```python
from build123d import *

# Parameters (mm, degrees)
ESQUISSE1_W              = 200
ESQUISSE1_H              = 200
BOSS_EXTRU_1_DEPTH       = 50
ESQUISSE2_W              = 190
ESQUISSE2_H              = 190
ENL_V_MAT_EXTRU_1_DEPTH  = 40
ESQUISSE3_W              = 70
ESQUISSE3_H              = 24
ENL_V_MAT_EXTRU_2_DEPTH  = 10
ESQUISSE5_W              = 5
ESQUISSE5_H              = 18
ESQUISSE5_W_2            = 30
ESQUISSE5_H_2            = 14
ENL_V_MAT_EXTRU_3_DEPTH  = 6
ESQUISSE7_W              = 5
ESQUISSE7_H              = 14
ENL_V_MAT_EXTRU_5_DEPTH  = 6
ESQUISSE8_W              = 80
ESQUISSE8_H              = 5
ENL_V_MAT_EXTRU_6_DEPTH  = 10
ESQUISSE9_W              = 190
ESQUISSE9_H              = 5
BOSS_EXTRU_2_DEPTH       = 75
ESQUISSE11_W             = 50
ESQUISSE11_H             = 40
ESQUISSE11_W_2           = 40
ESQUISSE11_H_2           = 30
ENL_V_MAT_EXTRU_9_DEPTH  = 6
ESQUISSE12_R             = 5.86708194
ENL_V_MAT_EXTRU_10_DEPTH = 2
ESQUISSE13_W             = 20
ESQUISSE13_H             = 10
ENL_V_MAT_EXTRU_11_DEPTH = 5


with BuildPart() as part:
    # Esquisse1 → Boss.-Extru.1 (new body)
    with BuildSketch(Plane(origin=(0, 0, 0), x_dir=(1, 0, 0), z_dir=(0, 1, 0))):
        Rectangle(ESQUISSE1_W, ESQUISSE1_H)
    extrude(amount=BOSS_EXTRU_1_DEPTH)

    # Esquisse2 → Enlèv. mat.-Extru.1 (cut)
    with BuildSketch(Plane.XZ):
        Rectangle(ESQUISSE2_W, ESQUISSE2_H)
    extrude(amount=-ENL_V_MAT_EXTRU_1_DEPTH, mode=Mode.SUBTRACT)

    # Esquisse3 → Enlèv. mat.-Extru.2 (cut)
    with BuildSketch(Plane(origin=(0, 50, 0), x_dir=(1, 0, 0), z_dir=(0, 1, 0))):
        with Locations((0, 72)):
            Rectangle(ESQUISSE3_W, ESQUISSE3_H)
    extrude(amount=-ENL_V_MAT_EXTRU_2_DEPTH, mode=Mode.SUBTRACT)

    # Esquisse5 → Enlèv. mat.-Extru.3 (cut)
    with BuildSketch(Plane.XZ.offset(-40)):
        with Locations((37.5, -72)):
            Rectangle(ESQUISSE5_W, ESQUISSE5_H)
        with Locations((-20, -53)):
            Rectangle(ESQUISSE5_W_2, ESQUISSE5_H_2)
    extrude(amount=-ENL_V_MAT_EXTRU_3_DEPTH, mode=Mode.SUBTRACT)

    # Esquisse7 → Enlèv. mat.-Extru.5 (cut)
    with BuildSketch(Plane.XZ.offset(-40)):
        with Locations((-37.5, -53)):
            Rectangle(ESQUISSE7_W, ESQUISSE7_H)
    extrude(amount=-ENL_V_MAT_EXTRU_5_DEPTH, mode=Mode.SUBTRACT)

    # Esquisse8 → Enlèv. mat.-Extru.6 (cut)
    with BuildSketch(Plane.XZ.offset(-40)):
        with Locations((0, -40)):
            Rectangle(ESQUISSE8_W, ESQUISSE8_H)
    extrude(amount=-ENL_V_MAT_EXTRU_6_DEPTH, mode=Mode.SUBTRACT)

    # Esquisse9 → Boss.-Extru.2 (add)
    with BuildSketch(Plane(origin=(0, 0, 95), x_dir=(-1, 0, 0), z_dir=(0, 0, -1))):
        with Locations((0, 2.5)):
            Rectangle(ESQUISSE9_W, ESQUISSE9_H)
    extrude(amount=BOSS_EXTRU_2_DEPTH)

    # Esquisse11 → Enlèv. mat.-Extru.9 (cut)
    with BuildSketch(Plane.XZ.offset(-40)):
        with Locations((0, 16)):
            Rectangle(ESQUISSE11_W, ESQUISSE11_H)
        with Locations((0, 16)):
            Rectangle(ESQUISSE11_W_2, ESQUISSE11_H_2, mode=Mode.SUBTRACT)
    extrude(amount=-ENL_V_MAT_EXTRU_9_DEPTH, mode=Mode.SUBTRACT)

    # Esquisse12 → Enlèv. mat.-Extru.10 (cut)
    with BuildSketch(Plane(origin=(0, 50, 0), x_dir=(1, 0, 0), z_dir=(0, 1, 0))):
        with Locations(Location((0, -14.714419725, 0), (0, 0, 270))):
            Circle(ESQUISSE12_R)
        with BuildLine():
            ThreePointArc((3.657276348, -2.723473664), (12.412554836, -14.744243454), (3.657276348, -26.765013245))
            ThreePointArc((3.657276348, -26.765013245), (3.359240733, -32.427689923), (9.021917411, -32.725725538))
            ThreePointArc((9.021917411, -32.725725538), (20.02990103, -14.744243454), (9.021917411, 3.237238629))
            ThreePointArc((9.021917411, 3.237238629), (3.359240733, 2.939203014), (3.657276348, -2.723473664))
        make_face()
        with BuildLine():
            ThreePointArc((-4.091649632, -2.723473664), (-12.057804345, -14.744243454), (-4.091649632, -26.765013245))
            ThreePointArc((-4.091649632, -26.765013245), (-4.087653986, -32.721729891), (-10.044370632, -32.725725538))
            ThreePointArc((-10.044370632, -32.725725538), (-20.198964068, -14.893261262), (-10.044370632, 2.939203014))
            ThreePointArc((-10.044370632, 2.939203014), (-4.236671793, 3.084225175), (-4.091649632, -2.723473664))
        make_face()
        with BuildLine():
            ThreePointArc((13.591796836, 10.19140297), (11.86542759, 15.688813034), (17.349999414, 17.455544504))
            ThreePointArc((17.349999414, 17.455544504), (36.455816795, -14.649786555), (17.402535548, -46.786323611))
            ThreePointArc((17.402535548, -46.786323611), (11.917488852, -45.152665208), (13.591796836, -39.679889879))
            ThreePointArc((13.591796836, -39.679889879), (27.918200585, -14.744243454), (13.591796836, 10.19140297))
        make_face()
        with BuildLine():
            ThreePointArc((-13.231408481, -39.679889879), (-12.247030277, -45.830218737), (-18.397359135, -46.814596942))
            ThreePointArc((-18.397359135, -46.814596942), (-36.414367356, -14.679352885), (-18.397359135, 17.455891172))
            ThreePointArc((-18.397359135, 17.455891172), (-12.182139707, 16.406622398), (-13.231408481, 10.19140297))
            ThreePointArc((-13.231408481, 10.19140297), (-28.157745811, -14.744243454), (-13.231408481, -39.679889879))
        make_face()
    extrude(amount=-ENL_V_MAT_EXTRU_10_DEPTH, mode=Mode.SUBTRACT)

    # Esquisse13 → Enlèv. mat.-Extru.11 (cut)
    with BuildSketch(Plane(origin=(-95, 0, 0), x_dir=(0, 0, -1), z_dir=(1, 0, 0))):
        with Locations((-30, 10)):
            Rectangle(ESQUISSE13_W, ESQUISSE13_H)
    extrude(amount=-ENL_V_MAT_EXTRU_11_DEPTH, mode=Mode.SUBTRACT)


solid = part.part
```
Input: part model. Units: mm. Frame: model coordinates. A direction names the side the tool comes from. Give positions to 0.01 mm unless a question says otherwise; leave off trailing zeros. Order: outer loops, then holes, each group sorted by start corner. A loop starts at its lowest first (then second) coordinate and runs counter-clockwise, first axis right, second up. Notation, with made-up numbers: M 25.25,12.5 L 57.25,12.5 A17 ccw 57.25,33.5 Z; hole C -3.5,12.5 d11. An arc over 180 degrees is marked long. Return JSON: item names as keys, results as strings.
1) Mould query, pull axis X, two halves, no side actions, for faces 1 (the face through (1, 0, 68)), 2 (the face through (-100, 25, 1)), 3 (the face through (-4.023, 49.014, 32.655)), 4 (the face through (100, 25, 1)). Classes: released by +X, released by -X, zero draft, split by the parting line, or undercut.
Taken from the geometry:
{"face 1": "zero draft", "face 2": "released by -X", "face 3": "undercut", "face 4": "released by +X"}
2) Section query D-D on z = -25. Output: boundary loops of the cut face in (x, y).
Taken from the geometry:
{"outline": "M -100,0 L -95,0 L -95,40 L 95,40 L 95,0 L 100,0 L 100,50 L -100,50 Z"}
3) Section query B-B on y = 31. Output: boundary loops of the cut face in (x, z).
Taken from the geometry:
{"outline": "M -100,-100 L 100,-100 L 100,100 L -100,100 Z; hole M -95,-95 L 95,-95 L 95,95 L -95,95 Z"}
4) Line query: L1, parallel to X at y = 14, z = 81; L2, parallel to Z at x = 69, y = 3.5. Output: solid intervals per line, ascending. Write a range as [from, to].
Taken from the geometry:
{"L1": "x = [-100, -95], [95, 100]", "L2": "z = [-100, -95], [20, 100]"}
5) Contact query for flat-ended pins moving along their axis: pin 1 (1 mm diameter, centred on x = 57, z = 38.5, fed in from -Y); pin 2 (10 mm diameter, centred on x = -25, z = -76, fed in from +Y). Output: stop coordinate, or through.
Taken from the geometry:
{"pin 1": "stops at y = 0", "pin 2": "passes through"}
6) Section query A-A on z = -70.5. Output: boundary loops of the cut face in (x, y), and give its area (3 significant figures).
Taken from the geometry:
{"outline": "M -100,0 L -95,0 L -95,40 L -35,40 L -35,50 L -100,50 Z; M 35,46 L 40,46 L 40,40 L 95,40 L 95,0 L 100,0 L 100,50 L 35,50 Z", "area": "1,670 mm2"}
7) Section query C-C on x = 0. Count the separate pieces of the cut face and the enclosed holes in it, and give its area (3 significant figures).
Taken from the geometry:
{"separate pieces": "3", "enclosed holes": "0", "area": "2,400 mm2"}
8) Access query for faces 5 (the face through (0, 43, -4)), 6 (the face through (-97, 10, 20)), 7 (the face through (0, 48, 15)), 8 (the face through (-95, 20, -1)). Directions: +Z, -Z, +X, -X, +Y, -Y. A direction counts if a zero-diameter tool reaches every point of the face in a straight line with its end or side. Return the directions, or none.
Taken from the geometry:
{"face 5": "-Y", "face 6": "-X", "face 7": "+Y", "face 8": "none"}
